Geometry check sheet. Reference: the model listing, model coordinates, mm. Face numbers are marked on the shaded views. A direction names the side the tool comes from. Round coordinates to 2 decimals unless told otherwise and drop trailing zeros. Order: outer loops, then holes, each group sorted by start corner. A loop starts at its lowest first (then second) coordinate and runs counter-clockwise, first axis right, second up.
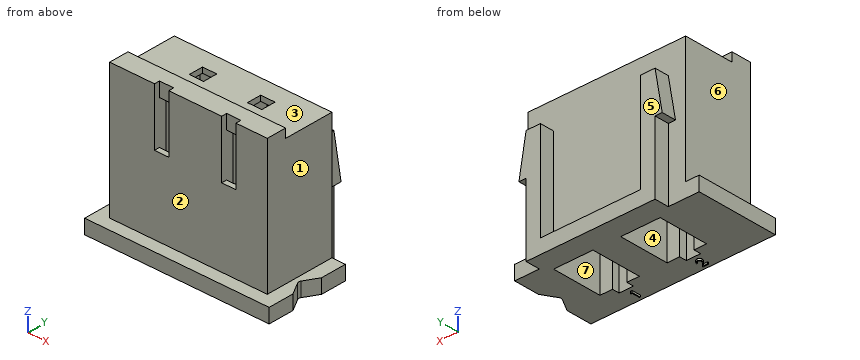
```python
from build123d import *

# Parameters (mm, degrees)
SKETCH1_W           = 8.8
SKETCH1_H           = 4.3
BOSS_EXTRUDE1_DEPTH = 7
SKETCH2_W           = 10.3
SKETCH2_H           = 4.6
BOSS_EXTRUDE2_DEPTH = 0.8
CUT_EXTRUDE1_DEPTH  = 1
FILLET1_R           = 0.2
SKETCH4_W           = 8.8
SKETCH4_H           = 1.5
BOSS_EXTRUDE3_DEPTH = 0.5
SKETCH5_W           = 0.8
SKETCH5_H           = 0.7
CUT_EXTRUDE2_DEPTH  = 3.2
SKETCH6_W           = 0.8
SKETCH6_H           = 0.8
CUT_EXTRUDE3_DEPTH  = 10
BOSS_EXTRUDE4_DEPTH = 0.8
CUT_EXTRUDE4_DEPTH  = 7.5
CUT_EXTRUDE5_DEPTH  = 0.4
BOSS_EXTRUDE5_DEPTH = 0.1


with BuildPart() as part:
    # Sketch1 → Boss-Extrude1 (new body)
    with BuildSketch(Plane.XY):
        Rectangle(SKETCH1_W, SKETCH1_H)
    extrude(amount=BOSS_EXTRUDE1_DEPTH)

    # Sketch2 → Boss-Extrude2 (add)
    with BuildSketch(Plane(origin=(0, 0, 0), x_dir=(-1, 0, 0), z_dir=(0, 0, -1))):
        with Locations((0, -0.15)):
            Rectangle(SKETCH2_W, SKETCH2_H)
    extrude(amount=BOSS_EXTRUDE2_DEPTH)

    # Sketch3 → Cut-Extrude1 (cut)
    with BuildSketch(Plane.XY):
        Polygon((4.65, -0.15), (5.15, -1.016025404), (5.15, 0.716025404), align=None)
    extrude(amount=-CUT_EXTRUDE1_DEPTH, mode=Mode.SUBTRACT)

    # Fillet1
    fillet1_edges = [part.edges().sort_by_distance(p)[0] for p in [
        (4.65, -0.15, -0.4),
    ]]
    fillet(fillet1_edges, radius=FILLET1_R)

    # Sketch4 → Boss-Extrude3 (add)
    with BuildSketch(Plane.XY.offset(7)):
        with Locations((0, -1.4)):
            Rectangle(SKETCH4_W, SKETCH4_H)
    extrude(amount=BOSS_EXTRUDE3_DEPTH)

    # Sketch5 → Cut-Extrude2 (cut)
    with BuildSketch(Plane.XY.offset(7.5)):
        with Locations((-1.5, -1.8)):
            Rectangle(SKETCH5_W, SKETCH5_H)
        with Locations((2.25, -1.8)):
            Rectangle(SKETCH5_W, SKETCH5_H)
    extrude(amount=-CUT_EXTRUDE2_DEPTH, mode=Mode.SUBTRACT)

    # Sketch6 → Cut-Extrude3 (cut)
    with BuildSketch(Plane.XY.offset(7)):
        with Locations((-1.5, 0.75)):
            Rectangle(SKETCH6_W, SKETCH6_H)
        with Locations((1.75, 0.75)):
            Rectangle(SKETCH6_W, SKETCH6_H)
    extrude(amount=-CUT_EXTRUDE3_DEPTH, mode=Mode.SUBTRACT)

    # Sketch7 → Boss-Extrude4 (add)
    with BuildSketch(Plane(origin=(0, 2.15, 0), x_dir=(1, 0, 0), z_dir=(0, 1, 0))):
        Polygon((-3.427970594, -5.5), (-3.827970594, -3.2), (-3.427970594, -3.2), (-3.427970594, 0.8), (3.772029406, 0.8), (3.772029406, -3.2), (4.172029406, -3.2), (3.772029406, -5.5), (2.972029406, -5.5), (2.972029406, 0), (-2.627970594, 0), (-2.627970594, -5.5), align=None)
    extrude(amount=BOSS_EXTRUDE4_DEPTH)

    # Sketch8 → Cut-Extrude4 (cut)
    with BuildSketch(Plane(origin=(0, 0, -0.8), x_dir=(-1, 0, 0), z_dir=(0, 0, -1))):
        Polygon((2.6, 1.746369259), (0.4, 1.746369259), (0.4, -1.053630741), (1.1, -1.053630741), (1.1, -1.453630741), (1.9, -1.453630741), (1.9, -1.053630741), (2.6, -1.053630741), align=None)
        Polygon((-1.15, 1.746369259), (-3.35, 1.746369259), (-3.35, -1.053630741), (-2.65, -1.053630741), (-2.65, -1.453630741), (-1.85, -1.453630741), (-1.85, -1.053630741), (-1.15, -1.053630741), align=None)
    extrude(amount=-CUT_EXTRUDE4_DEPTH, mode=Mode.SUBTRACT)

    # Sketch9 → Cut-Extrude5 (cut)
    with BuildSketch(Plane.XZ.offset(2.15)):
        Polygon((2.65, 7.5), (2.65, 4.3), (1.85, 4.3), (1.85, 7.5), (-1.1, 7.5), (-1.1, 4.3), (-1.9, 4.3), (-1.9, 7.5), (-4.4, 7.5), (-4.4, 0), (4.4, 0), (4.4, 7.5), align=None)
    extrude(amount=-CUT_EXTRUDE5_DEPTH, mode=Mode.SUBTRACT)

    # Sketch10 → Boss-Extrude5 (add)
    with BuildSketch(Plane(origin=(0, 0, -0.8), x_dir=(-1, 0, 0), z_dir=(0, 0, -1))):
        Polygon((-2.213189244, -1.663325944), (-2.120741327, -1.663325944), (-2.120741327, -2.163325944), (-2.165613122, -2.163325944), (-2.165613122, -1.714607995), (-2.242536199, -1.714607995), align=None)
        with BuildLine():
            Line((1.398489442, -1.817172097), (1.353617647, -1.817172097))
            add(Edge.make_bspline(
                [(1.353617647, -1.817172097), (1.353910097, -1.811219114), (1.354484462, -1.799527611), (1.357174218, -1.782481339), (1.361022915, -1.766187796), (1.366464551, -1.750777809), (1.373222591, -1.736115122), (1.38132688, -1.722257977), (1.390926002, -1.709259236), (1.401812678, -1.697239401), (1.413636769, -1.686212605), (1.426394761, -1.676690427), (1.439801193, -1.668645046), (1.453815393, -1.661919154), (1.468595473, -1.656870605), (1.48400731, -1.653124656), (1.500118616, -1.650870893), (1.511095762, -1.650628637), (1.516678544, -1.650505431)],
                knots=[0, 0, 0, 0, 1.7869e-05, 3.5094e-05, 5.1686e-05, 6.8032e-05, 8.4031e-05, 0.000100058, 0.000116104, 0.000132416, 0.000148647, 0.000164532, 0.000180078, 0.00019549, 0.000211074, 0.000226841, 0.000243017, 0.000259759, 0.000259759, 0.000259759, 0.000259759], degree=3))
            add(Edge.make_bspline(
                [(1.516678544, -1.650505431), (1.522161126, -1.650633782), (1.532934204, -1.650885987), (1.548657349, -1.653051848), (1.563625534, -1.656444075), (1.577809501, -1.661203421), (1.591096081, -1.667601196), (1.603585088, -1.675286559), (1.615425204, -1.684175106), (1.626083316, -1.694639936), (1.635870184, -1.705811706), (1.644313363, -1.717738549), (1.651543815, -1.730057018), (1.657570627, -1.742861047), (1.662007218, -1.756271194), (1.665375533, -1.770092223), (1.66727945, -1.784467196), (1.667571653, -1.794196704), (1.667720211, -1.799143251)],
                knots=[0, 0, 0, 0, 1.6441e-05, 3.2306e-05, 4.7516e-05, 6.2435e-05, 7.7085e-05, 9.1652e-05, 0.000106376, 0.000121393, 0.000136374, 0.000150882, 0.000165157, 0.000179183, 0.000193247, 0.000207458, 0.000221808, 0.000236648, 0.000236648, 0.000236648, 0.000236648], degree=3))
            add(Edge.make_bspline(
                [(1.667720211, -1.799143251), (1.667478316, -1.806107228), (1.666998772, -1.819912973), (1.662896718, -1.84020081), (1.656490074, -1.859857013), (1.648776166, -1.875676627), (1.640994388, -1.888424269), (1.633981887, -1.898919799), (1.625772628, -1.91022058), (1.616247128, -1.922288771), (1.605602432, -1.9352189), (1.593742123, -1.949003157), (1.580581626, -1.963499124), (1.571344697, -1.973399924), (1.566558352, -1.978530271)],
                knots=[0, 0, 0, 0, 2.0874e-05, 4.1382e-05, 6.1843e-05, 8.2763e-05, 9.3997e-05, 0.000106637, 0.000120621, 0.000135888, 0.000152753, 0.000170863, 0.000190435, 0.000211484, 0.000211484, 0.000211484, 0.000211484], degree=3))
            Line((1.566558352, -1.978530271), (1.441458192, -2.112043892))
            Line((1.441458192, -2.112043892), (1.674130467, -2.112043892))
            Line((1.674130467, -2.112043892), (1.674130467, -2.163325944))
            Line((1.674130467, -2.163325944), (1.334386878, -2.163325944))
            Line((1.334386878, -2.163325944), (1.528297134, -1.956394854))
            add(Edge.make_bspline(
                [(1.528297134, -1.956394854), (1.533018261, -1.951466524), (1.542086579, -1.942000212), (1.554912661, -1.928179789), (1.566432517, -1.915358426), (1.576720716, -1.903560348), (1.585554074, -1.892612981), (1.593392964, -1.88287088), (1.599673763, -1.873905959), (1.606490248, -1.863514443), (1.613092245, -1.850826969), (1.618765439, -1.835322156), (1.622224703, -1.81936112), (1.622639679, -1.808575115), (1.622848416, -1.803149662)],
                knots=[0, 0, 0, 0, 2.0474e-05, 3.9327e-05, 5.6561e-05, 7.2184e-05, 8.6278e-05, 9.8762e-05, 0.000109683, 0.000119101, 0.000136035, 0.000152448, 0.000168517, 0.00018478, 0.00018478, 0.00018478, 0.00018478], degree=3))
            add(Edge.make_bspline(
                [(1.622848416, -1.803149662), (1.622757596, -1.799738033), (1.622578606, -1.793014369), (1.620998935, -1.783156403), (1.61861172, -1.773647144), (1.615190969, -1.764457341), (1.61067572, -1.755679391), (1.605179523, -1.747302608), (1.598838086, -1.739204185), (1.59150219, -1.731610856), (1.583443402, -1.724656398), (1.574929937, -1.718495815), (1.56592278, -1.71334737), (1.556459905, -1.709126871), (1.546567695, -1.705816102), (1.536227017, -1.703522019), (1.525466443, -1.702081664), (1.518118801, -1.701886783), (1.514374859, -1.701787482)],
                knots=[0, 0, 0, 0, 1.0229e-05, 2.0159e-05, 2.9876e-05, 3.9606e-05, 4.9505e-05, 5.9423e-05, 6.9622e-05, 8.0319e-05, 9.1042e-05, 0.000101521, 0.000111795, 0.000122107, 0.000132559, 0.000143032, 0.000153841, 0.00016507, 0.00016507, 0.00016507, 0.00016507], degree=3))
            add(Edge.make_bspline(
                [(1.514374859, -1.701787482), (1.51046474, -1.70188963), (1.502785912, -1.70209023), (1.491511764, -1.703493468), (1.480756653, -1.705914302), (1.470493524, -1.709225256), (1.460705012, -1.71343362), (1.45143872, -1.718675298), (1.44271545, -1.724930083), (1.434518804, -1.732021591), (1.426966807, -1.739916962), (1.420331539, -1.748718385), (1.414533822, -1.758265159), (1.40947536, -1.768531523), (1.405367405, -1.779610635), (1.402228383, -1.791463164), (1.399744548, -1.804037647), (1.398914759, -1.812721231), (1.398489442, -1.817172097)],
                knots=[0, 0, 0, 0, 1.1729e-05, 2.3035e-05, 3.4018e-05, 4.4756e-05, 5.5343e-05, 6.5928e-05, 7.6628e-05, 8.7492e-05, 9.8403e-05, 0.00010934, 0.000120489, 0.000131867, 0.000143625, 0.00015587, 0.000168619, 0.000182025, 0.000182025, 0.000182025, 0.000182025], degree=3))
        make_face()
    extrude(amount=BOSS_EXTRUDE5_DEPTH)


solid = part.part
```
(1) Sectioned sample at D-D, the plane y = 2.6. Record the cut outline in (x, z), and give its area (3 significant figures).
Returned:
outline: (-3.83, 3.2) - (-3.43, 3.2) - (-3.43, -0.8) - (3.77, -0.8) - (3.77, 3.2) - (4.17, 3.2) - (3.77, 5.5) - (2.97, 5.5) - (2.97, 0) - (-2.63, 0) - (-2.63, 5.5) - (-3.43, 5.5) - close
area: 15.5 mm2
(2) Set-up check for the marked faces 1, 2 and 3: record each of +Z, -Z, +X, -X, +Y, -Y from which the full face is reachable in a straight line by a thin tool's end or side.
Returned:
face 1: +Z, +X, +Y, -Y
face 2: +Z, +X, -X, -Y
face 3: +Z, +X, -X, +Y
(3) Sectioned sample at C-C, the plane y = 0.9. Record the cut outline in (x, z), and give its area (3 significant figures).
Returned:
outline: (-5.15, -0.8) - (-2.6, -0.8) - (-2.6, 6.7) - (-1.9, 6.7) - (-1.9, 7) - (-4.4, 7) - (-4.4, 0) - (-5.15, 0) - close; (-1.1, 6.7) - (-0.4, 6.7) - (-0.4, -0.8) - (1.15, -0.8) - (1.15, 6.7) - (1.35, 6.7) - (1.35, 7) - (-1.1, 7) - close; (2.15, 6.7) - (3.35, 6.7) - (3.35, -0.8) - (5.15, -0.8) - (5.15, 0) - (4.4, 0) - (4.4, 7) - (2.15, 7) - close
area: 36.4 mm2
(4) Depth check by flat-ended pin: P1, Ø1.4, axis at x = 2, y = 0.5, coming from the +Z side; P2, Ø2, axis at y = 0.5, z = 4.5, coming from the +X side; P3, Ø0.6, axis at y = -1.5, z = 5, coming from the -X side. Enter the tip coordinate at first touch or a pass-through.
Returned:
P1: stops at z = 7
P2: stops at x = 4.4
P3: stops at x = -4.4
(5) Draft check along X on the marked faces 4, 5, 6 and 7. Enter one of: released by +X, released by -X, zero draft, split by the parting line, or undercut.
Returned:
face 4: undercut
face 5: zero draft
face 6: released by -X
face 7: undercut
(6) Material ranges on line 1 (X direction, y = 0.25, z = 4.5); line 2 (Y direction, x = 2, z = 1.5); line 3 (Y direction, x = -0.5, z = 4), recorded low to high.
Returned:
line 1: x = -4.4 to -2.6, -0.4 to 1.15, 3.35 to 4.4
line 2: y = -1.75 to -1.45, 1.75 to 2.15
line 3: y = -1.75 to -1.05, 1.75 to 2.15
(7) Sectioned sample at B-B, the plane z = -0.5. Record the cut outline in (x, y), and give its area (3 significant figures).
Returned:
outline: (-5.15, -2.45) - (5.15, -2.45) - (5.15, -1.02) - (4.71, -0.25) arc R0.2 cw to (4.71, -0.05) - (5.15, 0.72) - (5.15, 2.15) - (3.77, 2.15) - (3.77, 2.95) - (-3.43, 2.95) - (-3.43, 2.15) - (-5.15, 2.15) - close; hole (-2.6, -1.05) - (-1.9, -1.05) - (-1.9, -1.45) - (-1.1, -1.45) - (-1.1, -1.05) - (-0.4, -1.05) - (-0.4, 1.75) - (-2.6, 1.75) - close; hole (1.15, -1.05) - (1.85, -1.05) - (1.85, -1.45) - (2.65, -1.45) - (2.65, -1.05) - (3.35, -1.05) - (3.35, 1.75) - (1.15, 1.75) - close
area: 39.7 mm2
(8) Sectioned sample at A-A, the plane x = 2.5. Record the cut outline in (y, z).
Returned:
outline: (-2.45, -0.8) - (-1.45, -0.8) - (-1.45, 4.3) - (-1.75, 4.3) - (-1.75, 0) - (-2.45, 0) - close; (-1.45, 6.7) - (1.75, 6.7) - (1.75, -0.8) - (2.95, -0.8) - (2.95, 0) - (2.15, 0) - (2.15, 7) - (-0.65, 7) - (-0.65, 7.5) - (-1.45, 7.5) - close
